```python
from build123d import *

# Parameters (mm, degrees)
SKETCH1_R           = 15
BOSS_EXTRUDE1_DEPTH = 60
SKETCH2_W           = 50
SKETCH2_H           = 50
CUT_EXTRUDE1_DEPTH  = 120


with BuildPart() as part:
    # Sketch1 → Boss-Extrude1 (new body, symmetric)
    with BuildSketch(Plane.XY):
        with BuildLine():
            Line((30, -60), (40, -60))
            Line((40, -60), (40, -43.369403571))
            Line((40, -43.369403571), (60, -43.369403571))
            Line((60, -43.369403571), (60, 42.942577675))
            Line((60, 42.942577675), (40, 42.942577675))
            Line((40, 42.942577675), (40, 60))
            Line((40, 60), (12.5, 60))
            ThreePointArc((12.5, 60), (0, 47.5), (-12.5, 60))
            Line((-12.5, 60), (-40, 60))
            Line((-40, 60), (-40, 42.942577675))
            Line((-40, 42.942577675), (-60, 42.942577675))
            Line((-60, 42.942577675), (-60, 0))
            Line((-60, 0), (-60, -43.369403571))
            Line((-60, -43.369403571), (-40, -43.369403571))
            Line((-40, -43.369403571), (-40, -60))
            Line((-40, -60), (-30, -60))
            ThreePointArc((-30, -60), (0, -30), (30, -60))
        make_face()
        Circle(SKETCH1_R, mode=Mode.SUBTRACT)
    extrude(amount=BOSS_EXTRUDE1_DEPTH, both=True)

    # Sketch2 → Cut-Extrude1 (cut)
    with BuildSketch(Plane(origin=(60, 0, 0), x_dir=(0, 0, -1), z_dir=(1, 0, 0))):
        Rectangle(SKETCH2_W, SKETCH2_H)
    extrude(amount=-CUT_EXTRUDE1_DEPTH, mode=Mode.SUBTRACT)


solid = part.part
```
The listing builds one solid part. Answer for the finished solid, in the listing's coordinates (mm). A direction names the side the tool comes from. Give positions to 0.01 mm unless a question says otherwise; leave off trailing zeros. Loops run counter-clockwise (first coordinate to the right, second up) from the corner with the lowest first, then second, coordinate; pieces in that order, holes last. Notation, with made-up numbers: M -14.75,29 L 21.25,29 A28 cw 21.25,67 Z; hole C -20,55 d11. An arc over 180 degrees is marked long. One line per item, written item: value.
Q1. Determine the mould class of faces 5 (the face through (12, 14, -60)), 6 (the face through (50, -43.369, 1)), 7 (the face through (1, -25, 0)), 8 (the face through (14, -6, 25)) for opening direction Z: +Z half, -Z half, draft (parallel to the pull), parting line (faces both ways), or undercut.
Working result:
face 5: -Z half
face 6: draft
face 7: undercut
face 8: undercut
Q2. A cutting plane is placed at A-A on y = 0. Determine the outline of the cut face in (x, z), then the cut area to 3 significant figures.
Working result:
outline: M -60,-60 L -15,-60 L -15,-25 L -60,-25 Z; M -60,25 L -15,25 L -15,60 L -60,60 Z; M 15,-60 L 60,-60 L 60,-25 L 15,-25 Z; M 15,25 L 60,25 L 60,60 L 15,60 Z
area: 6,300 mm^2
Q3. Find the intervals of material crossed by line 1 (Y direction, x = 0, z = 44); line 2 (X direction, y = 0, z = 35.5); line 3 (Z direction, x = -17, y = 7.5), in increasing order. Write a range as from..to.
Working result:
line 1: y = -30..-15, 15..47.5
line 2: x = -60..-15, 15..60
line 3: z = -60..-25, 25..60
Q4. A cutting plane is placed at B-B on x = 45.5. Determine the outline of the cut face in (y, z), then the cut area to 3 significant figures.
Working result:
outline: M -43.37,-60 L 42.94,-60 L 42.94,60 L -43.37,60 Z; hole M -25,-25 L 25,-25 L 25,25 L -25,25 Z
area: 7,860 mm^2
Q5. A cutting plane is placed at D-D on y = 23. Determine the outline of the cut face in (x, z), then the cut area to 3 significant figures.
Working result:
outline: M -60,-60 L 60,-60 L 60,-25 L -60,-25 Z; M -60,25 L 60,25 L 60,60 L -60,60 Z
area: 8,400 mm^2
Q6. For faces 1 (the face through (1, 25, 0)), 2 (the face through (40, 51, 1)), 3 (the face through (-50, 42.943, 1)), 4 (the face through (-40, -52, 1)), determine the directions among +Z, -Z, +X, -X, +Y, -Y from which every point of the face is accessible in a straight line to the end or side of a thin tool.
Working result:
face 1: +X, -X
face 2: +Z, -Z, +X, +Y
face 3: +Z, -Z, -X, +Y
face 4: +Z, -Z, -X, -Y
Q7. Flat-ended cylindrical pins translate along their axes: P1, Ø5, axis at y = -55, z = -5.5, coming from the -X side; P2, Ø12, axis at x = -3.5, z = 28, coming from the -Y side; P3, Ø6, axis at x = -52.5, z = 9.5, coming from the +Y side; P4, Ø15, axis at x = 0, y = -8, coming from the -Z side. Find the tip coordinate at first contact, or state that the pin passes through.
Working result:
P1: stops at x = -40
P2: stops at y = -31.54
P3: stops at y = 42.94
P4: stops at z = -60
Q8. A cutting plane is placed at C-C on z = -43. Determine the outline of the cut face in (x, y).
Working result:
outline: M -60,-43.37 L -40,-43.37 L -40,-60 L -30,-60 A30 cw 30,-60 L 40,-60 L 40,-43.37 L 60,-43.37 L 60,42.94 L 40,42.94 L 40,60 L 12.5,60 A12.5 cw -12.5,60 L -40,60 L -40,42.94 L -60,42.94 Z; hole C 0,0 d30
